Geometry check sheet. Reference: drawing and pictorial views, mm from the part's lowest x, y, z. A direction names the side the tool comes from. Round coordinates to 2 decimals unless told otherwise and drop trailing zeros. Order: outer loops, then holes, each group sorted by start corner. A loop starts at its lowest first (then second) coordinate and runs counter-clockwise, first axis right, second up. Notation, with made-up numbers: M -18,52 L 24,52 A12 ccw 24,65 Z; hole C 80.25,-28.5 d9. An arc over 180 degrees is marked long. Answer as a JSON object with one key per item and string values. Group by question number.
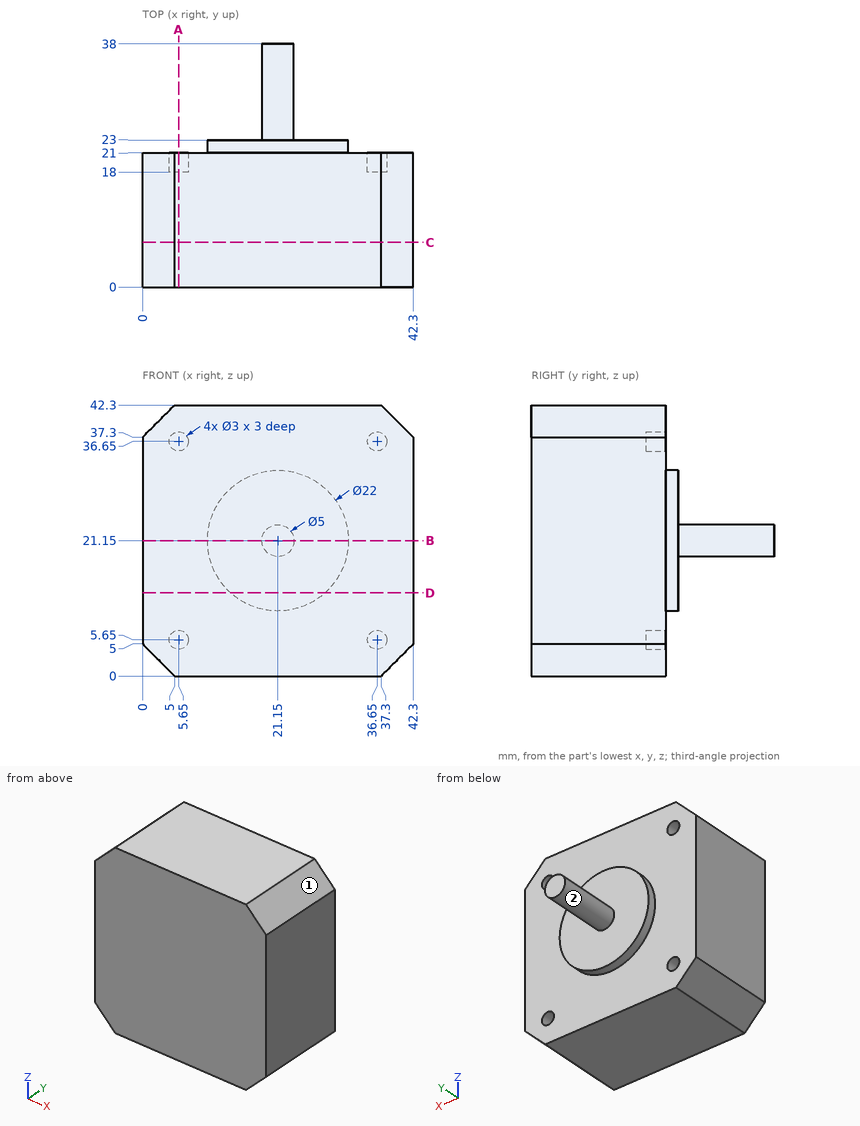
Q1. Tool access check on the marked faces 1 and 2. Record the directions out of +Z, -Z, +X, -X, +Y, -Y that give a thin tool (end or side, any length) a straight path to the whole face; none if there is none.
Q2. Cross-section at A-A, the plane x = 5.65. Record the cut outline in (y, z).
Q3. Gauge pin test, flat ends, axial feed: pin 1 Ø3 at (x, z) = (13, 4.5) entering from -Y; pin 2 Ø1.5 at (x, z) = (21.5, 15) entering from +Y; pin 3 Ø5 at (x, z) = (36.65, 5.65) entering from +Y; pin 4 Ø2.5 at (x, z) = (5.5, 5.5) entering from +Y. Record the tip position at first contact, or that the pin passes through.
Q4. Cross-section at D-D, the plane z = 13. Record the cut outline in (x, y), then the cut area to 3 significant figures.
Q5. Cross-section at C-C, the plane y = 7. Record the cut outline in (x, z).
Q6. Thickness scan on line 1 (Z direction, x = 5.5, y = 20); line 2 (X direction, y = 19, z = 5); line 3 (Y direction, x = 4, z = 19.5). Record the ranges inside material, lowest first. Write a range as from..to.
Q7. Cross-section at B-B, the plane z = 21.15. Record the cut outline in (x, y), then the cut area to 3 significant figures.
Conclusion:
{
 "1": {"face 1": "+Z, +X, +Y, -Y", "face 2": "+Y"},
 "2": {"outline": "M 0,0 L 21,0 L 21,4.15 L 18,4.15 L 18,7.15 L 21,7.15 L 21,35.15 L 18,35.15 L 18,38.15 L 21,38.15 L 21,42.3 L 0,42.3 Z"},
 "3": {"pin 1": "y = 0", "pin 2": "y = 23", "pin 3": "y = 21", "pin 4": "y = 18"},
 "4": {"outline": "M 0,0 L 42.3,0 L 42.3,21 L 28.54,21 L 28.54,23 L 13.76,23 L 13.76,21 L 0,21 Z", "area": "918 mm2"},
 "5": {"outline": "M 0,5 L 5,0 L 37.3,0 L 42.3,5 L 42.3,37.3 L 37.3,42.3 L 5,42.3 L 0,37.3 Z"},
 "6": {"line 1": "0..4.16, 7.14..35.16, 38.14..42.3", "line 2": "0..4.3, 7..35.3, 38..42.3", "line 3": "0..21"},
 "7": {"outline": "M 0,0 L 42.3,0 L 42.3,21 L 32.15,21 L 32.15,23 L 23.65,23 L 23.65,38 L 18.65,38 L 18.65,23 L 10.15,23 L 10.15,21 L 0,21 Z", "area": "1,010 mm2"}
}
